from build123d import *

# Parameters (mm, degrees)
BASPROSKE_W         = 12.7
BASPROSKE_H         = 13.97
TOOTHCUT_DEPTH      = 24.486417351
TEETHCUTS_COUNT     = 20
HUBNEAONESKE_R      = 6.35
HUBNEARONE_DEPTH    = 6.3502032
BORSKE_R            = 3.175
BORE_DEPTH          = 19.0502032
SKETCH1_R           = 3.175
BOSS_EXTRUDE1_DEPTH = 19.0502032
SKETCH2_R           = 7.9375
CUT_EXTRUDE1_DEPTH  = 5.08


with BuildPart() as part:
    # BasProSke → Base-Revolve (revolve)
    with BuildSketch(Plane(origin=(0, 0, 0), x_dir=(1, 0, 0), z_dir=(0, 1, 0)), mode=Mode.PRIVATE) as base_revolve_sk:
        with Locations((6.35, 6.985)):
            Rectangle(BASPROSKE_W, BASPROSKE_H)
    revolve(base_revolve_sk.sketch.rotate(Axis((-10, 0, 0), (1, 0, 0)), 180), axis=Axis((-10, 0, 0), (1, 0, 0)))

    # TooCutSke → ToothCut (cut, through all)
    with BuildSketch(Plane(origin=(0, 0, 0), x_dir=(0, 0, -1), z_dir=(1, 0, 0))):
        with BuildLine():
            ThreePointArc((0.64046545, 11.106749257), (0, 11.1252), (-0.64046545, 11.106749257))
            ThreePointArc((-0.64046545, 11.106749257), (-1.052455812, 12.582227662), (-1.8855699, 13.867798935))
            ThreePointArc((-1.8855699, 13.867798935), (0, 13.9954), (1.8855699, 13.867798935))
            ThreePointArc((1.8855699, 13.867798935), (1.052455812, 12.582227662), (0.64046545, 11.106749257))
        make_face()
    toothcut = extrude(amount=TOOTHCUT_DEPTH, mode=Mode.SUBTRACT)

    # TeethCuts: ToothCut ×20 about axis
    teethcuts_axis = Axis((-10, 0, 0), (1, 0, 0))
    for i in range(1, TEETHCUTS_COUNT):
        add(toothcut.rotate(teethcuts_axis, i * 360 / TEETHCUTS_COUNT), mode=Mode.SUBTRACT)

    # HubNeaOneSke → HubNearOne (add)
    with BuildSketch(Plane.ZY):
        with Locations(Location((0, 0, 0), (0, 0, 180))):
            Circle(HUBNEAONESKE_R)
    extrude(amount=HUBNEARONE_DEPTH)

    # BorSke → Bore (cut, symmetric)
    with BuildSketch(Plane(origin=(0, 0, 0), x_dir=(0, 0, -1), z_dir=(1, 0, 0))):
        with Locations(Location((0, 0, 0), (0, 0, 180))):
            Circle(BORSKE_R)
    extrude(amount=BORE_DEPTH, both=True, mode=Mode.SUBTRACT)

    # Sketch1 → Boss-Extrude1 (add)
    with BuildSketch(Plane.ZY.offset(6.3502032)):
        Circle(SKETCH1_R)
        with BuildLine():
            Line((-2, 2.236067977), (-2, -2.236067977))
            ThreePointArc((-2, -2.236067977), (3, 0), (-2, 2.236067977))
        make_face(mode=Mode.SUBTRACT)
    extrude(amount=-BOSS_EXTRUDE1_DEPTH)

    # Sketch2 → Cut-Extrude1 (cut)
    with BuildSketch(Plane(origin=(12.7, 0, 0), x_dir=(0, 0, -1), z_dir=(1, 0, 0))):
        Circle(SKETCH2_R)
    extrude(amount=-CUT_EXTRUDE1_DEPTH, mode=Mode.SUBTRACT)


solid = part.part
For this review, take the finished solid that the model builds, in its own axes (mm). A direction names the side the tool comes from. Give positions to 0.01 mm unless a question says otherwise; leave off trailing zeros. Loops run counter-clockwise (first coordinate to the right, second up) from the corner with the lowest first, then second, coordinate; pieces in that order, holes last. Notation, with made-up numbers: M 58.25,58.25 L 64.25,58.25 A30 ccw 64.25,80.25 Z; hole C 69,9 d1. An arc over 180 degrees is marked long. Put each result on its own line as item: value. Start each with the question number.
(1) Add section C-C, the plane x = -3.5. Write out the cut boundary in (y, z), then the cut area to 4 significant figures.
(2) For pin 1 (8 mm diameter, centred on x = 7, y = 3, fed in from -Z); pin 2 (1.5 mm diameter, centred on y = -1.5, z = -8, fed in from -X); pin 3 (8 mm diameter, centred on x = 4.5, y = 9.5, fed in from +Z), all flat-tipped, find the tip position at first contact; note any pin that passes through.
(3) Machinability: for faces 1 (the cylindrical face through (6.261, -8.215, 9.542)), 2 (the cylindrical face through (6.261, 11.646, -4.893)), 3 (the cylindrical face through (6.261, -12.298, -2.887)), which of the approach directions +Z, -Z, +X, -X, +Y, -Y give a long, thin tool a straight path to every point of the face, cutting with its end or side? Answer none if there is none.
(4) Add section B-B, the plane z = 0. Write out the cut boundary in (x, y).
(5) Add section A-A, the plane y = 0. Write out the cut boundary in (x, z).
(6) The part is to be moulded in two halves that separate along Y. For faces 4 (the cylindrical face through (6.261, -9.542, -8.215)), 5 (the cylindrical face through (6.261, -1.055, -12.588)), 6 (the cylindrical face through (6.261, 3.446, 10.578)), 7 (the cylindrical face through (6.261, 12.588, -1.055)), say which applies: +Y half, -Y half, draft (parallel to the pull), parting line (faces both ways), or undercut.
(7) Add section D-D, the plane z = 5. Write out the cut boundary in (x, y), then the cut area to 3 significant figures.
(8) Wall thickness on L1, parallel to Y at x = 6.75, z = 11.5; L2, parallel to Z at x = 6.5, y = -12; L3, parallel to Y at x = -2.5, z = 0: over which ranges is each line inside the solid? List them lowest first.
Result:
1. outline: C 0,0 d12.7; hole M -2.24,-2 L 2.24,-2 A3 ccw long Z
1. area: 101.5 mm^2
2. pin 1: stops at z = -13.84
2. pin 2: stops at x = 0
2. pin 3: stops at z = 12.59
3. face 1: +Z, +X, -X
3. face 2: +X, -X, +Y
3. face 3: +X, -X
4. outline: M -6.35,-6.35 L 0,-6.35 L 0,-11.13 L 12.7,-11.13 L 12.7,-7.94 L 7.62,-7.94 L 7.62,-3 L -6.35,-3 Z; M -6.35,3 L 7.62,3 L 7.62,7.94 L 12.7,7.94 L 12.7,11.13 L 0,11.13 L 0,6.35 L -6.35,6.35 Z
5. outline: M -6.35,-6.35 L 0,-6.35 L 0,-11.13 L 12.7,-11.13 L 12.7,-7.94 L 7.62,-7.94 L 7.62,-2 L -6.35,-2 Z; M -6.35,3 L 7.62,3 L 7.62,7.94 L 12.7,7.94 L 12.7,11.13 L 0,11.13 L 0,6.35 L -6.35,6.35 Z
6. face 4: -Y half
6. face 5: undercut
6. face 6: undercut
6. face 7: +Y half
7. outline: M -6.35,-3.91 L 0,-3.91 L 0,-11.76 L 12.7,-11.76 L 12.7,-6.16 L 7.62,-6.16 L 7.62,6.16 L 12.7,6.16 L 12.7,11.76 L 0,11.76 L 0,3.91 L -6.35,3.91 Z
7. area: 286 mm^2
8. L1: y = -6.64 to -4.77, -2.91 to -0.7, 0.7 to 2.91, 4.77 to 6.64
8. L2: z = -6.65 to -5.25, -2.91 to -0.83, 0.83 to 2.91, 5.25 to 6.65
8. L3: y = -6.35 to -3, 3 to 6.35
